Part model, mm, in its own coordinate system. Face numbers are marked on the shaded views. A direction names the side the tool comes from. Give positions to 0.01 mm unless a question says otherwise; leave off trailing zeros. Write each loop counter-clockwise with the first axis right and the second up, starting at its lowest first coordinate (ties: lowest second). Pieces come first, ordered by that corner, then holes. Notation, with made-up numbers: (37.5, 72) - (51.5, 72) arc R27 ccw to (51.5, 91) - close; hole circle Ø4 at (-16, -21). An arc over 180 degrees is marked (long way). Answer in a Markdown table with one row per item. Add a question column.
1. Band-saw the part on C-C on z = 16. Write the cut outline in (x, y), plus the area to 3 significant figures.
2. Drop flat-ended pins along their axis: pin 1 Ø16 at (x, z) = (65.5, 23.5) entering from +Y; pin 2 Ø2 at (x, z) = (17, 40) entering from +Y. Give the stop position or say it passes through.
3. Which spindle directions (+Z, -Z, +X, -X, +Y, -Y) get a long thin tool onto all of the face, cutting with end or side? Do the marked faces 4 and 5. Say none if no direction does.
4. Band-saw the part on B-B on x = 45.5. Write the cut outline in (y, z), plus the area to 3 significant figures.
5. Probe line 1 along X through (y, z) = (58, 29.5); line 2 along Z through (x, y) = (55, 53); line 3 along Y through (x, z) = (122.5, 13.5). List the from-to ranges inside material, lowest first.
6. Pull direction X, two halves, no side cores. Call the marked faces 1, 2 and 3: released by +X, released by -X, zero draft, split by the parting line, or undercut.
7. Band-saw the part on A-A on y = 25.5. Write the cut outline in (x, z).
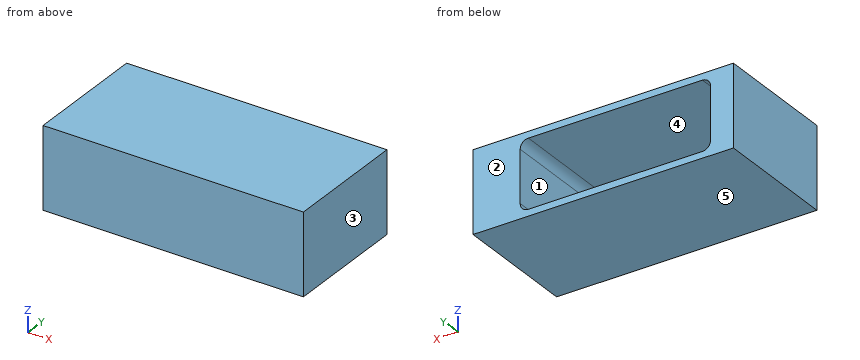
Autodesk Fusion 360 part; units mm, degrees
sketch "Esboço1" plane through (0, 0, 0) normal (0, 1, 0) x (1, 0, 0)
  line L0 (0, 0) -> (160, 0)
  line L1 (160, 0) -> (160, -50)
  line L2 (160, -50) -> (0, -50)
  line L3 (0, -50) -> (0, 0)
  dimension "d1" = 160
  dimension "d2" = 50
extrude "Extrusão1" add sketch "Esboço1" along normal blind 77
sketch "Esboço2" plane through (0, 77, 0) normal (0, 1, 0) x (-1, 0, 0)
  line L0 (0, 50) -> (-160, 50)
  line L1 (-160, 50) -> (-160, 0)
  line L2 (-160, 0) -> (0, 0)
  line L3 (0, 0) -> (0, 50)
  line L4 (-131, 46) -> (-14, 46)
  line L5 (-14, 46) -> (-14, 4)
  line L6 (-14, 4) -> (-131, 4)
  line L7 (-131, 4) -> (-131, 46)
  dimension "d5" = 117
  dimension "d6" = 42
  dimension "d7" = 4
  dimension "d8" = 4
  dimension "d9" = 14
extrude "Extrusão2" cut sketch "Esboço2" against normal blind 75 contours L4 L5 L6 L7
fillet "Arredondamento1" radius 5 8 edges at (14, 2, 25) (14, 39.5, 4) (14, 39.5, 46) (72.5, 2, 4) (131, 39.5, 4) (131, 2, 25) (72.5, 2, 46) (131, 39.5, 46)
Values:
| question | item | result |
|---|---|---|
| 1 | outline | (0, 0) - (160, 0) - (160, 77) - (131, 77) - (131, 7) arc R5 cw to (126, 2) - (19, 2) arc R5 cw to (14, 7) - (14, 77) - (0, 77) - close |
| 1 | area | 3,560 mm² |
| 2 | pin 1 | stops at y = 2 |
| 2 | pin 2 | stops at y = 3 |
| 3 | face 4 | +Y |
| 3 | face 5 | -Z, +X, -X, +Y, -Y |
| 4 | outline | (0, 0) - (77, 0) - (77, 4) - (7, 4) arc R5 cw to (2, 9) - (2, 41) arc R5 cw to (7, 46) - (77, 46) - (77, 50) - (0, 50) - close |
| 4 | area | 711 mm² |
| 5 | line 1 | x = 0 to 14, 131 to 160 |
| 5 | line 2 | z = 0 to 4, 46 to 50 |
| 5 | line 3 | y = 0 to 2 |
| 6 | face 1 | undercut |
| 6 | face 2 | zero draft |
| 6 | face 3 | released by +X |
| 7 | outline | (0, 0) - (160, 0) - (160, 50) - (0, 50) - close; hole (14, 9) arc R5 ccw to (19, 4) - (126, 4) arc R5 ccw to (131, 9) - (131, 41) arc R5 ccw to (126, 46) - (19, 46) arc R5 ccw to (14, 41) - close |
